```python
from build123d import *

# Parameters (mm, degrees)
SKETCH_1_W      = 38
SKETCH_1_H      = 38
SKETCH_1_R      = 2.5
SKETCH_1_R_2    = 6
EXTRUDE_1_DEPTH = 9
FILLET_1_R      = 5


with BuildPart() as part:
    # 草图1 → 凸台-拉伸1 (new body)
    with BuildSketch(Plane.XY):
        with Locations((-2.169799589, 0.839779006)):
            Rectangle(SKETCH_1_W, SKETCH_1_H)
        with Locations((8.830200411, 11.839779006)):
            Circle(SKETCH_1_R, mode=Mode.SUBTRACT)
        with Locations((8.830200411, -10.160220994)):
            Circle(SKETCH_1_R, mode=Mode.SUBTRACT)
        with Locations((-13.169799589, -10.160220994)):
            Circle(SKETCH_1_R, mode=Mode.SUBTRACT)
        with Locations((-6.169799589, 4.839779006)):
            Circle(SKETCH_1_R_2, mode=Mode.SUBTRACT)
    extrude(amount=EXTRUDE_1_DEPTH)

    # 圆角1
    fillet_1_edges = [part.edges().sort_by_distance(p)[0] for p in [
        (-21.169799589, 19.839779006, 4.5),
        (16.830200411, 19.839779006, 4.5),
        (16.830200411, -18.160220994, 4.5),
        (-21.169799589, -18.160220994, 4.5),
    ]]
    fillet(fillet_1_edges, radius=FILLET_1_R)


solid = part.part
```
For this review, take the finished solid that the model builds, in its own axes (mm). Give positions to 0.01 mm unless a question says otherwise; leave off trailing zeros. Order: outer loops, then holes, each group sorted by start corner. A loop starts at its lowest first (then second) coordinate and runs counter-clockwise, first axis right, second up.
1) Take a section at D-D (y = 4). Give the boundary of the cut face in (x, z).
2) Insertion check: pin 1 (6 mm diameter, centred on x = 8.83, y = 11.84, fed in from +Z); pin 2 (4.5 mm diameter, centred on x = 8.83, y = -10.16, fed in from +Z). Each pin has a flat end and moves straight along its axis. Give the tip position at first contact, or say it passes through.
3) Wall thickness on line 1 (Y direction, x = 9, z = 3.25); line 2 (Y direction, x = 11, z = 8.75); line 3 (X direction, y = 10, z = 8.25): over which ranges is each line inside the solid? List them lowest first.
4) Take a section at B-B (z = 4.25). Give the boundary of the cut face in (x, y).
5) Take a section at A-A (y = -11.5). Give the boundary of the cut face in (x, z), then the cut area to 3 significant figures.
6) The part is to be moulded in two halves that separate along Y. For faces 1 (the face through (-10.93, 1.19, 4.44)), 2 (the face through (6.99, -8.47, 4.44)), 3 (the face through (-19.7, -16.7, 4.6)), 4 (the face through (15.33, 18.41, 4.56)), say which applies: released by +Y, released by -Y, zero draft, split by the parting line, or undercut.
7) Take a section at C-C (x = -9.5). Give the boundary of the cut face in (y, z), then the cut area to 3 significant figures.
Derived:
1. outline: (-21.17, 0) - (-12.11, 0) - (-12.11, 9) - (-21.17, 9) - close; (-0.23, 0) - (16.83, 0) - (16.83, 9) - (-0.23, 9) - close
2. pin 1: stops at z = 9
2. pin 2: passes through
3. line 1: y = -18.16 to -12.65, -7.67 to 9.35, 14.33 to 19.84
3. line 2: y = -18.16 to -11.4, -8.92 to 10.6, 13.08 to 19.84
3. line 3: x = -21.17 to -9.23, -3.11 to 7.14, 10.52 to 16.83
4. outline: (-21.17, -13.16) arc R5 ccw to (-16.17, -18.16) - (11.83, -18.16) arc R5 ccw to (16.83, -13.16) - (16.83, 14.84) arc R5 ccw to (11.83, 19.84) - (-16.17, 19.84) arc R5 ccw to (-21.17, 14.84) - close; hole circle Ø5 at (-13.17, -10.16); hole circle Ø12 at (-6.17, 4.84); hole circle Ø5 at (8.83, -10.16); hole circle Ø5 at (8.83, 11.84)
5. outline: (-21.17, 0) - (-15.28, 0) - (-15.28, 9) - (-21.17, 9) - close; (-11.06, 0) - (6.72, 0) - (6.72, 9) - (-11.06, 9) - close; (10.94, 0) - (16.83, 0) - (16.83, 9) - (10.94, 9) - close
5. area: 266 mm2
6. face 1: undercut
6. face 2: undercut
6. face 3: released by -Y
6. face 4: released by +Y
7. outline: (-18.16, 0) - (-0.15, 0) - (-0.15, 9) - (-18.16, 9) - close; (9.83, 0) - (19.84, 0) - (19.84, 9) - (9.83, 9) - close
7. area: 252 mm2
